For this review, take the finished solid that the model builds, in its own axes (mm). A direction names the side the tool comes from. Give positions to 0.01 mm unless a question says otherwise; leave off trailing zeros. Order: outer loops, then holes, each group sorted by start corner. A loop starts at its lowest first (then second) coordinate and runs counter-clockwise, first axis right, second up. Notation, with made-up numbers: (-3, 83.25) - (38, 83.25) arc R14 ccw to (38, 109.25) - close; hole circle Ø7 at (-7, -24.75). An arc over 180 degrees is marked (long way). Use a Markdown table: item, result. Add a question column.
1) We need section A-A on y = 0. Write out the cut boundary in (x, z).
2) Machinability: for faces 1 (the face through (-1.437, 1.318, 6.535)), 2 (the face through (0, 2.95, -4)), 3 (the face through (-1, 2, 9)), which of the approach directions +Z, -Z, +X, -X, +Y, -Y give a long, thin tool a straight path to every point of the face, cutting with its end or side? Answer none if there is none.
3) Clearance check with flat-ended pins moving along their axes: P1, Ø2, axis at y = -1, z = 5.5, coming from the +X side; P2, Ø0.5, axis at x = 2.5, z = 2.5, coming from the -Y side; P3, Ø1.5, axis at x = 4.5, y = 1, coming from the -Z side. State where each tip first meets the part, or that it passes through.
4) We need section C-C on x = 0. Write out the cut boundary in (y, z), then the cut area to 3 significant figures.
5) Wall thickness on L1, parallel to Y at x = -4.5, z = -2.25; L2, parallel to Y at x = 0, z = 6.15; L3, parallel to Z at x = 2, y = -2.75: over which ranges is each line inside the solid? List them lowest first.
6) We need section D-D on z = 2.75. Write out the cut boundary in (x, y).
7) We need section B-B on z = -2.25. Write out the cut boundary in (x, y).
8) Mouldability with a two-part tool opening along X and no side actions: class faces 4 (the face through (2.45, 0, 5)), 5 (the face through (0, 0, 4)), 6 (the face through (0, 0, -0.3)) as released by +X, released by -X, zero draft, split by the parting line, or undercut.
```python
from build123d import *

# Parameters (mm, degrees)
SKETCH005_W     = 12.9
SKETCH005_H     = 5.9
PAD003_DEPTH    = 0.3
FILLET003_R     = 1
SKETCH006_W     = 9.8
SKETCH006_H     = 0.3
PAD004_DEPTH    = 8.55
PAD005_DEPTH    = 0.3
FILLET004_R     = 0.3
SKETCH008_R     = 2.9
PAD006_DEPTH    = 9
SKETCH009_R     = 1.95
POCKET002_DEPTH = 5
CHAMFER_SIZE    = 0.5
SKETCH010_W     = 0.5
SKETCH010_H     = 0.8
POCKET003_DEPTH = 9


with BuildPart() as part:
    # Sketch005 → Pad003 (new body)
    with BuildSketch(Plane.XY):
        Rectangle(SKETCH005_W, SKETCH005_H)
    extrude(amount=-PAD003_DEPTH)

    # Fillet003
    fillet003_edges = [part.edges().sort_by_distance(p)[0] for p in [
        (-6.45, -2.95, -0.15),
        (-6.45, 2.95, -0.15),
        (6.45, 2.95, -0.15),
        (6.45, -2.95, -0.15),
    ]]
    fillet(fillet003_edges, radius=FILLET003_R)

    # Sketch006 (on Face2 of Fillet003) → Pad004 (join)
    with BuildSketch(Plane.XY):
        with Locations((0, 3.1)):
            Rectangle(SKETCH006_W, SKETCH006_H)
        with Locations((0, -3.1)):
            Rectangle(SKETCH006_W, SKETCH006_H)
    extrude(amount=-PAD004_DEPTH)

    # Sketch007 (on Face21 of Pad004) → Pad005 (join)
    with BuildSketch(Plane(origin=(0, 0, -8.55), x_dir=(1, 0, 0), z_dir=(0, 0, -1))):
        with BuildLine():
            ThreePointArc((-3.05, 2.95), (-2.3, 2.2), (-1.55, 2.95))
            Line((-1.55, 2.95), (-1.55, 3.25))
            Line((-3.05, 3.25), (-1.55, 3.25))
            Line((-3.05, 3.25), (-3.05, 2.95))
        make_face()
        with BuildLine():
            ThreePointArc((1.55, 2.95), (2.3, 2.2), (3.05, 2.95))
            Line((3.05, 2.95), (3.05, 3.25))
            Line((1.55, 3.25), (3.05, 3.25))
            Line((1.55, 3.25), (1.55, 2.95))
        make_face()
        with BuildLine():
            ThreePointArc((-1.55, -2.95), (-2.3, -2.2), (-3.05, -2.95))
            Line((-3.05, -2.95), (-3.05, -3.25))
            Line((-3.05, -3.25), (-1.55, -3.25))
            Line((-1.55, -3.25), (-1.55, -2.95))
        make_face()
        with BuildLine():
            ThreePointArc((3.05, -2.95), (2.3, -2.2), (1.55, -2.95))
            Line((1.55, -2.95), (1.55, -3.25))
            Line((1.55, -3.25), (3.05, -3.25))
            Line((3.05, -3.25), (3.05, -2.95))
        make_face()
    extrude(amount=PAD005_DEPTH)

    # Fillet004
    fillet004_edges = [part.edges().sort_by_distance(p)[0] for p in [
        (-2.3, -3.25, -8.85),
        (2.3, -3.25, -8.85),
        (2.3, 3.25, -8.85),
        (-2.3, 3.25, -8.85),
        (0, 3.25, 0),
        (0, -3.25, 0),
    ]]
    fillet(fillet004_edges, radius=FILLET004_R)

    # Sketch008 (on Face1 of Fillet004) → Pad006 (join)
    with BuildSketch(Plane.XY):
        Circle(SKETCH008_R)
    extrude(amount=PAD006_DEPTH)

    # Sketch009 (on Face22 of Pad006) → Pocket002 (cut)
    with BuildSketch(Plane.XY.offset(9)):
        Circle(SKETCH009_R)
    extrude(amount=-POCKET002_DEPTH, mode=Mode.SUBTRACT)

    # Chamfer
    chamfer_edges = [part.edges().sort_by_distance(p)[0] for p in [
        (-2.9, 0, 9),
    ]]
    chamfer(chamfer_edges, length=CHAMFER_SIZE)

    # Sketch010 (on Face4 of Chamfer) → Pocket003 (cut)
    with BuildSketch(Plane.XY.offset(9)):
        with Locations((2.7, 0)):
            Rectangle(SKETCH010_W, SKETCH010_H)
    extrude(amount=-POCKET003_DEPTH, mode=Mode.SUBTRACT)


solid = part.part
```
Checked values:
| question | item | result |
|---|---|---|
| 1 | outline | (-6.45, -0.3) - (6.45, -0.3) - (6.45, 0) - (2.45, 0) - (2.45, 8.95) - (2.4, 9) - (1.95, 9) - (1.95, 4) - (-1.95, 4) - (-1.95, 9) - (-2.4, 9) - (-2.9, 8.5) - (-2.9, 0) - (-6.45, 0) - close |
| 2 | face 1 | +Z |
| 2 | face 2 | +X, -X |
| 2 | face 3 | +Z, +X, -X, +Y, -Y |
| 3 | P1 | x = 2.87 |
| 3 | P2 | y = -1.83 |
| 3 | P3 | z = -0.3 |
| 4 | outline | (-3.25, -8.55) - (-2.95, -8.55) - (-2.95, -0.3) - (2.95, -0.3) - (2.95, -8.55) - (3.25, -8.55) - (3.25, -0.3) arc R0.3 ccw to (2.95, 0) - (2.9, 0) - (2.9, 8.5) - (2.4, 9) - (1.95, 9) - (1.95, 4) - (-1.95, 4) - (-1.95, 9) - (-2.4, 9) - (-2.9, 8.5) - (-2.9, 0) - (-2.95, 0) arc R0.3 ccw to (-3.25, -0.3) - close |
| 4 | area | 39.3 mm² |
| 5 | L1 | -3.25 to -2.95, 2.95 to 3.25 |
| 5 | L2 | -2.9 to -1.95, 1.95 to 2.9 |
| 5 | L3 | -8.85 to -8.55, -0.3 to 0 |
| 6 | outline | (2.45, -0.4) - (2.45, 0.4) - (2.87, 0.4) arc R2.9 ccw (long way) to (2.87, -0.4) - close |
| 7 | outline | (-4.9, -3.25) - (4.9, -3.25) - (4.9, -2.95) - (-4.9, -2.95) - close; (-4.9, 2.95) - (4.9, 2.95) - (4.9, 3.25) - (-4.9, 3.25) - close |
| 8 | face 4 | released by +X |
| 8 | face 5 | undercut |
| 8 | face 6 | zero draft |
